Geometry: final body of the model. Coordinates: model frame, mm. Give positions to 0.01 mm unless a question says otherwise; leave off trailing zeros. Loops run counter-clockwise (first coordinate to the right, second up) from the corner with the lowest first, then second, coordinate; pieces in that order, holes last. Notation, with made-up numbers: (-16.75, 24) -> (15.25, 24) arc R28 ccw to (15.25, 52) -> close; hole circle Ø4 at (55.5, 40). An arc over 180 degrees is marked (long way). Answer in a Markdown table with one row per item. Add a question column.
1) Section query A-A (y = 0.85). Return the cut outline in (x, z).
2) Line query: line 1 (X direction, y = 0.3, z = 2.25); line 2 (X direction, y = 0.6, z = 1.75); line 3 (Z direction, x = -1, y = 0.9). Output: solid intervals per line, ascending. Write a range as from..to.
3) Section query B-B (x = -25). Return the cut outline in (y, z).
4) Section query C-C (z = -3.25). Return the cut outline in (x, y).
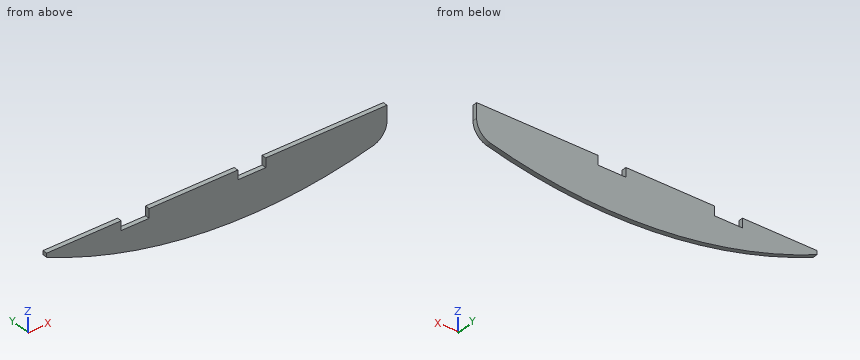
```python
from build123d import *

# Parameters (mm, degrees)
EXTRUDE_1_DEPTH     = 1
SKETCH_2_W          = 6
SKETCH_2_H          = 4
CUT_EXTRUDE_1_DEPTH = 2
FILLET_1_R          = 4


with BuildPart() as part:
    # 草图1 → 凸台-拉伸1 (new body)
    with BuildSketch(Plane(origin=(0, 0, 0), x_dir=(1, 0, 0), z_dir=(0, 1, 0))):
        with BuildLine():
            Line((-30, -3), (-44, -3))
            Line((-44, -3), (-44, -2.158291102))
            ThreePointArc((-44, -2.158291102), (-7.97872831, 6.982895336), (29, 3.286010669))
            Line((29, 3.286010669), (29, -3))
            Line((29, -3), (0, -3))
            Line((0, -3), (-30, -3))
        make_face()
    extrude(amount=EXTRUDE_1_DEPTH)

    # 草图2 → 切除-拉伸1 (cut, through all)
    with BuildSketch(Plane.XZ):
        with Locations((0, 3)):
            Rectangle(SKETCH_2_W, SKETCH_2_H)
        with Locations((-25, 3)):
            Rectangle(SKETCH_2_W, SKETCH_2_H)
    extrude(amount=-CUT_EXTRUDE_1_DEPTH, mode=Mode.SUBTRACT)

    # 圆角1
    fillet_1_edges = [part.edges().sort_by_distance(p)[0] for p in [
        (29, 0.5, -3.286010669),
    ]]
    fillet(fillet_1_edges, radius=FILLET_1_R)


solid = part.part
```
Evaluation:
| question | item | result |
|---|---|---|
| 1 | outline | (-44, 2.16) arc R107.28 ccw to (25.97, -4.09) arc R4 ccw to (29, -0.21) -> (29, 3) -> (3, 3) -> (3, 1) -> (-3, 1) -> (-3, 3) -> (-22, 3) -> (-22, 1) -> (-28, 1) -> (-28, 3) -> (-44, 3) -> close |
| 2 | line 1 | -44..-28, -22..-3, 3..29 |
| 2 | line 2 | -43.08..-28, -22..-3, 3..29 |
| 2 | line 3 | -7.28..1 |
| 3 | outline | (0, -4.33) -> (1, -4.33) -> (1, 1) -> (0, 1) -> close |
| 4 | outline | (-29.13, 0) -> (27.6, 0) -> (27.6, 1) -> (-29.13, 1) -> close |
